Verification items for the finished model (mm, model axes). A direction names the side the tool comes from. Round coordinates to 2 decimals unless told otherwise and drop trailing zeros. Order: outer loops, then holes, each group sorted by start corner. A loop starts at its lowest first (then second) coordinate and runs counter-clockwise, first axis right, second up. Notation, with made-up numbers: M 52,-30 L 106,-30 A28 cw 106,3 Z; hole C 55,88.5 d4. An arc over 180 degrees is marked long. Return JSON: item names as keys, results as strings. Group by question number.
from build123d import *

# Parameters (mm, degrees)
AUFSATZ_LINEAR_AUSTRAGEN1_DEPTH = 25
SKIZZE2_W                       = 6
SKIZZE2_H                       = 1.8
AUFSATZ_LINEAR_AUSTRAGEN2_DEPTH = 8
SKIZZE3_W                       = 7.5
SKIZZE3_H                       = 0.4
SCHNITT_LINEAR_AUSTRAGEN1_DEPTH = 34
VERRUNDUNG1_R                   = 0.2


with BuildPart() as part:
    # Skizze1 → Aufsatz-Linear austragen1 (new body)
    with BuildSketch(Plane.XY):
        Polygon((-4.75, 0.9), (-6.7, 0.9), (-6.7, -0.9), (-4.75, -0.9), (-4.75, -2.9), (-3.75, -2.9), (-3.75, -0.9), (3.75, -0.9), (3.75, -2.9), (4.75, -2.9), (4.75, -0.9), (6.7, -0.9), (6.7, 0.9), (4.75, 0.9), (4.75, 2.9), (3.75, 2.9), (3.75, 0.9), (-3.75, 0.9), (-3.75, 2.9), (-4.75, 2.9), align=None)
    extrude(amount=AUFSATZ_LINEAR_AUSTRAGEN1_DEPTH)

    # Skizze2 → Aufsatz-Linear austragen2 (add)
    with BuildSketch(Plane(origin=(0, 0, 0), x_dir=(-1, 0, 0), z_dir=(0, 0, -1))):
        Rectangle(SKIZZE2_W, SKIZZE2_H)
    extrude(amount=AUFSATZ_LINEAR_AUSTRAGEN2_DEPTH)

    # Skizze3 → Schnitt-Linear austragen1 (cut, through all)
    with BuildSketch(Plane.XY.offset(25)):
        with Locations((0, -0.7)):
            Rectangle(SKIZZE3_W, SKIZZE3_H)
        with Locations((0, 0.7)):
            Rectangle(SKIZZE3_W, SKIZZE3_H)
    extrude(amount=-SCHNITT_LINEAR_AUSTRAGEN1_DEPTH, mode=Mode.SUBTRACT)

    # Verrundung1
    verrundung1_edges = [part.edges().sort_by_distance(p)[0] for p in [
        (0, 0.5, 25),
        (-4.75, -1.9, 25),
        (-4.25, -2.9, 25),
        (-5.725, 0.9, 0),
        (-4.75, 1.9, 0),
        (-4.25, 2.9, 0),
        (-3.75, -1.7, 25),
        (4.25, 2.9, 0),
        (4.75, 1.9, 0),
        (5.725, 0.9, 0),
        (6.7, 0, 0),
        (5.725, -0.9, 0),
        (4.75, -1.9, 0),
        (4.25, -2.9, 0),
        (-4.25, -2.9, 0),
        (-4.75, -1.9, 0),
        (-5.725, -0.9, 0),
        (-6.7, 0, 0),
        (3.75, -1.7, 25),
        (4.25, -2.9, 25),
        (-6.7, 0.9, 12.5),
        (-4.75, 2.9, 12.5),
        (-3.75, 2.9, 12.5),
        (3.75, 2.9, 12.5),
        (4.75, 2.9, 12.5),
        (6.7, 0.9, 12.5),
        (6.7, -0.9, 12.5),
        (4.75, -2.9, 12.5),
        (3.75, -2.9, 12.5),
        (-3.75, -2.9, 12.5),
        (-4.75, -2.9, 12.5),
        (-6.7, -0.9, 12.5),
        (4.75, -1.9, 25),
        (5.725, -0.9, 25),
        (6.7, 0, 25),
        (5.725, 0.9, 25),
        (-6.7, 0, 25),
        (4.75, 1.9, 25),
        (4.25, 2.9, 25),
        (3.75, 1.7, 25),
        (-3.75, 1.7, 25),
        (3, 0, -8),
        (-3, 0, -8),
        (-4.25, 2.9, 25),
        (0, 0.5, -8),
        (0, -0.5, -8),
        (-4.75, 1.9, 25),
        (-5.725, 0.9, 25),
        (0, -0.5, 25),
        (-5.725, -0.9, 25),
    ]]
    fillet(verrundung1_edges, radius=VERRUNDUNG1_R)


solid = part.part
1. Cross-section at C-C (x = -0.75). Enter the section's corners in (y, z), plus the area to 3 significant figures.
2. Access from +Z, -Z, +X, -X, +Y, -Y to the whole of each face (thin tool, end or side, straight path). Record for faces 1 (the face through (-6, -0.9, 12)), 2 (the face through (0, 0.5, 9)), 3 (the face through (-3.75, -2, 13)).
3. Draft check along X on faces 4 (the face through (5, 0, 0)), 5 (the face through (-3, 0, -4)), 6 (the face through (0, -0.5, 9)). Enter one of: +X half, -X half, draft (parallel to the pull), parting line (faces both ways), or undercut.
4. Cross-section at A-A (y = -1.9). Enter the section's corners in (x, z), plus the area to 3 significant figures.
5. Thickness scan on line 1 along X through (y, z) = (-1.4, 12.5); line 2 along X through (y, z) = (-0.7, 6); line 3 along Y through (x, z) = (3.5, 20). Record the ranges inside material, lowest first. Write a range as from..to.
6. Go/stop test with flat-tipped pins: pin 1 (0.5 mm diameter, centred on y = 0, z = -2.5, fed in from -X); pin 2 (1.5 mm diameter, centred on x = 0, z = 8.5, fed in from -Y); pin 3 (2 mm diameter, centred on x = 3, y = -2, fed in from -Z). Record where each tip stops, or that it passes through.
7. Cross-section at D-D (x = -5.5). Enter the section's corners in (y, z), plus the area to 3 significant figures.
Computed:
{
 "1": {"outline": "M -0.5,-7.8 A0.2 ccw -0.3,-8 L 0.3,-8 A0.2 ccw 0.5,-7.8 L 0.5,24.8 A0.2 ccw 0.3,25 L -0.3,25 A0.2 ccw -0.5,24.8 Z", "area": "33.0 mm²"},
 "2": {"face 1": "+Z, -Z, -X, -Y", "face 2": "+Z, -Z, +Y", "face 3": "+Z, -Z, -Y"},
 "3": {"face 4": "draft", "face 5": "-X half", "face 6": "undercut"},
 "4": {"outline": "M -4.75,0.2 A0.2 ccw -4.55,0 L -3.75,0 L -3.75,24.8 A0.2 ccw -3.95,25 L -4.55,25 A0.2 ccw -4.75,24.8 Z; M 3.75,0 L 4.55,0 A0.2 ccw 4.75,0.2 L 4.75,24.8 A0.2 ccw 4.55,25 L 3.95,25 A0.2 ccw 3.75,24.8 Z", "area": "49.9 mm²"},
 "5": {"line 1": "x = -4.75..-3.75, 3.75..4.75", "line 2": "x = -6.7..-3.75, 3.75..6.7", "line 3": "y = -0.5..0.5"},
 "6": {"pin 1": "stops at x = -3", "pin 2": "stops at y = -0.5", "pin 3": "stops at z = 0"},
 "7": {"outline": "M -0.9,0.2 A0.2 ccw -0.7,0 L 0.7,0 A0.2 ccw 0.9,0.2 L 0.9,24.8 A0.2 ccw 0.7,25 L -0.7,25 A0.2 ccw -0.9,24.8 Z", "area": "45.0 mm²"}
}
